Geometry: final body of the model. Coordinates: model frame, mm. Face numbers are marked on the shaded views. A direction names the side the tool comes from. Give positions to 0.01 mm unless a question says otherwise; leave off trailing zeros. Loops run counter-clockwise (first coordinate to the right, second up) from the corner with the lowest first, then second, coordinate; pieces in that order, holes last. Notation, with made-up numbers: (85.5, 45) -> (123.5, 45) arc R18 cw to (123.5, 64) -> close; hole circle Ø11 at (53, 49.5). An arc over 180 degrees is marked (long way). Answer in a Markdown table with one row per item. Add a question column.
1) First-contact query: P1, Ø1.5, axis at x = 0, z = 1.5, coming from the +Y side; P2, Ø2, axis at x = 1, y = 7.5, coming from the +Z side. Flat tips, straight axial feed; report the tip coordinate or a pass-through.
2) Section query A-A (y = 5.25). Return the cut outline in (x, z).
3) Draft query along Z for the marked faces 3, 4 and 5. Return one class per face: +Z half, -Z half, draft (parallel to the pull), parting line (faces both ways), or undercut.
4) Access query for the marked faces 1 and 2. Directions: +Z, -Z, +X, -X, +Y, -Y. A direction counts if a zero-diameter tool reaches every point of the face in a straight line with its end or side. Return the directions, or none.
5) Line query: line 1 (Z direction, x = -0.45, y = 10.75); line 2 (X direction, y = 2, z = 0.2); line 3 (Y direction, x = 1.1, z = -0.1). Output: solid intervals per line, ascending. Write a range as from..to.
```python
from build123d import *

# Parameters (mm, degrees)
SKETCH_1_R          = 1
EXTRUDE_1_DEPTH     = 10
SKETCH_2_R          = 2
EXTRUDE_2_DEPTH     = 1.5
CUT_EXTRUDE_1_DEPTH = 1


with BuildPart() as part:
    # 草图1 → 凸台-拉伸1 (new body)
    with BuildSketch(Plane(origin=(0, 0, 0), x_dir=(1, 0, 0), z_dir=(0, 1, 0))):
        Circle(SKETCH_1_R)
    extrude(amount=EXTRUDE_1_DEPTH)

    # 草图2 → 凸台-拉伸2 (add)
    with BuildSketch(Plane(origin=(0, 10, 0), x_dir=(1, 0, 0), z_dir=(0, 1, 0))):
        Circle(SKETCH_2_R)
    extrude(amount=EXTRUDE_2_DEPTH)

    # 草图3 → 切除-拉伸1 (cut)
    with BuildSketch(Plane(origin=(0, 11.5, 0), x_dir=(1, 0, 0), z_dir=(0, 1, 0))):
        Polygon((0.609304592, -0.615424987), (0.837625969, 0.219960762), (0.228321377, 0.835385749), (-0.609304592, 0.615424987), (-0.837625969, -0.219960762), (-0.228321377, -0.835385749), align=None)
    extrude(amount=-CUT_EXTRUDE_1_DEPTH, mode=Mode.SUBTRACT)

    # 草图5 → 切除-旋转4 (revolve, cut)
    with BuildSketch(Plane.XY):
        with BuildLine():
            add(Edge.make_bspline(
                [(-0.5, 11.452368755), (-2, 11.161895004), (-2, 10)],
                knots=[4.965069236, 4.965069236, 4.965069236, 6.283185307, 6.283185307, 6.283185307], degree=2, weights=[1, 0.790569415, 1]))
            Line((-2, 10), (-2, 11.5))
            Line((-2, 11.5), (-0.5, 11.5))
            Line((-0.5, 11.5), (-0.5, 11.452368755))
        make_face()
    revolve(axis=Axis((0, 11.5, 0), (0, -1, 0)), mode=Mode.SUBTRACT)


solid = part.part
```
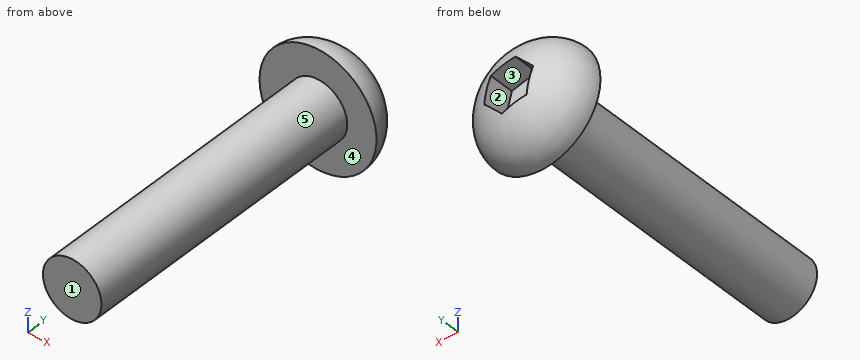
Evaluation:
| question | item | result |
|---|---|---|
| 1 | P1 | y = 11.39 |
| 1 | P2 | z = 1 |
| 2 | outline | circle Ø2 at (0, 0) |
| 3 | face 3 | undercut |
| 3 | face 4 | draft |
| 3 | face 5 | parting line |
| 4 | face 1 | +Z, -Z, +X, -X, -Y |
| 4 | face 2 | +Y |
| 5 | line 1 | -1.67..-0.66, 0.61..1.67 |
| 5 | line 2 | -0.98..0.98 |
| 5 | line 3 | 10..11.25 |
